from build123d import *

# Parameters (mm, degrees)
SKETCH1_W           = 50
SKETCH1_H           = 36
SKETCH1_R           = 8
SKETCH1_W_2         = 11.807071599
SKETCH1_H_2         = 5.093325141
BOSS_EXTRUDE1_DEPTH = 3
SKETCH2_W           = 50
SKETCH2_H           = 18
SKETCH2_R           = 1.6
BOSS_EXTRUDE2_DEPTH = 3
FILLET1_R           = 5
FILLET2_R           = 2


with BuildPart() as part:
    # Sketch1 → Boss-Extrude1 (new body)
    with BuildSketch(Plane.XY):
        with Locations((0, 18)):
            Rectangle(SKETCH1_W, SKETCH1_H)
        with Locations((-13, 20)):
            Circle(SKETCH1_R, mode=Mode.SUBTRACT)
        with Locations((14.084852814, 20)):
            Circle(SKETCH1_R, mode=Mode.SUBTRACT)
        with Locations((0.491645941, 27.45333743)):
            Rectangle(SKETCH1_W_2, SKETCH1_H_2, mode=Mode.SUBTRACT)
    extrude(amount=BOSS_EXTRUDE1_DEPTH)

    # Sketch2 → Boss-Extrude2 (add)
    with BuildSketch(Plane(origin=(0, 0, 0), x_dir=(1, 0, 0), z_dir=(0, 1, 0))):
        with Locations((0, 6)):
            Rectangle(SKETCH2_W, SKETCH2_H)
        with Locations(Location((0, 7.5, 0), (0, 0, 270))):
            Circle(SKETCH2_R, mode=Mode.SUBTRACT)
        with Locations(Location((-11, 7.5, 0), (0, 0, 270))):
            Circle(SKETCH2_R, mode=Mode.SUBTRACT)
        with Locations(Location((11, 7.5, 0), (0, 0, 270))):
            Circle(SKETCH2_R, mode=Mode.SUBTRACT)
    extrude(amount=BOSS_EXTRUDE2_DEPTH)

    # Fillet1
    fillet1_edges = [part.edges().sort_by_distance(p)[0] for p in [
        (-25, 1.5, -15),
        (25, 1.5, -15),
        (-25, 36, 1.5),
        (25, 36, 1.5),
    ]]
    fillet(fillet1_edges, radius=FILLET1_R)

    # Fillet2
    fillet2_edges = [part.edges().sort_by_distance(p)[0] for p in [
        (0, 3, 0),
        (0, 0, 3),
    ]]
    fillet(fillet2_edges, radius=FILLET2_R)


solid = part.part
Can you work these out from the model? Positions are in its coordinate system, mm. A direction names the side the tool comes from. Give positions to 0.01 mm unless a question says otherwise; leave off trailing zeros. Loops run counter-clockwise (first coordinate to the right, second up) from the corner with the lowest first, then second, coordinate; pieces in that order, holes last. Notation, with made-up numbers: (54.5, 31) -> (67.5, 31) arc R16 cw to (67.5, 37) -> close; hole circle Ø2 at (74.5, 88). An arc over 180 degrees is marked (long way). Use one line per item in the form item = value.
1) We'd pull the mould along X, two halves only. Please class faces 1 (the face through (24, 2, -13)), 2 (the face through (0, 19, 3)), 3 (the face through (-14.041, 27.932, 1.479)): released by +X, released by -X, zero draft, split by the parting line, or undercut.
Answers:
face_1 = released by +X
face_2 = zero draft
face_3 = undercut
2) For faces 4 (the face through (0, 24.907, 1)), 5 (the face through (0, 21, 0)), 6 (the face through (0, 0, -5)), which set-ups out of +Z, -Z, +X, -X, +Y, -Y let a thin tool reach every point of the face, with its end or its side?
Answers:
face_4 = +Z, -Z
face_5 = -Z, +X, -X, +Y
face_6 = +Z, -Z, +X, -X, -Y
3) If we section it at A-A (x = 0): Please give me the cut outline in (y, z), plus the area to 3 significant figures.
Answers:
outline = (0, -15) -> (3, -15) -> (3, -9.1) -> (0, -9.1) -> close; (0, -5.9) -> (3, -5.9) -> (3, -2) arc R2 cw to (5, 0) -> (24.91, 0) -> (24.91, 3) -> (2, 3) arc R2 ccw to (0, 1) -> close; (30, 0) -> (36, 0) -> (36, 3) -> (30, 3) -> close
area = 128 mm²
4) If we section it at B-B (y = 20): Please give me the cut outline in (x, z).
Answers:
outline = (-25, 0) -> (-21, 0) -> (-21, 3) -> (-25, 3) -> close; (-5, 0) -> (6.08, 0) -> (6.08, 3) -> (-5, 3) -> close; (22.08, 0) -> (25, 0) -> (25, 3) -> (22.08, 3) -> close
5) I need wall thicknesses on line 1 along X through (y, z) = (2, -7.5); line 2 along Y through (x, z) = (-13, 0.9); line 3 along Z through (x, y) = (9, 26.5). Which ranges of each line are inside material? Lowest first, please.
Answers:
line_1 = -25 to -12.6, -9.4 to -1.6, 1.6 to 9.4, 12.6 to 25
line_2 = 0 to 12, 28 to 36
line_3 = 0 to 3
6) If we section it at D-D (x = 14): Please give me the cut outline in (y, z), plus the area to 3 significant figures.
Answers:
outline = (0, -15) -> (3, -15) -> (3, -2) arc R2 cw to (5, 0) -> (12, 0) -> (12, 3) -> (2, 3) arc R2 ccw to (0, 1) -> close; (28, 0) -> (36, 0) -> (36, 3) -> (28, 3) -> close
area = 105 mm²
7) Will this pin go through, and if not, where does the flat tip stop? pin 1 (15.5 mm diameter, centred on x = 1.5, y = 19, fed in from -Z).
Answers:
pin_1 = 0
8) If we section it at C-C (y = 26): Please give me the cut outline in (x, z).
Answers:
outline = (-25, 0) -> (-18.29, 0) -> (-18.29, 3) -> (-25, 3) -> close; (-7.71, 0) -> (-5.41, 0) -> (-5.41, 3) -> (-7.71, 3) -> close; (6.4, 0) -> (8.79, 0) -> (8.79, 3) -> (6.4, 3) -> close; (19.38, 0) -> (25, 0) -> (25, 3) -> (19.38, 3) -> close
